Read the model definition and answer for the solid it produces. Units are mm, in the model's axes. Give positions to 0.01 mm unless a question says otherwise; leave off trailing zeros. Order: outer loops, then holes, each group sorted by start corner. A loop starts at its lowest first (then second) coordinate and runs counter-clockwise, first axis right, second up. Notation, with made-up numbers: (-34.75, 83.5) - (-5.75, 83.5) arc R7 cw to (-5.75, 91.5) - close; hole circle Ø7 at (-2, 30). An arc over 180 degrees is marked (long way). Write item = value, one per line.
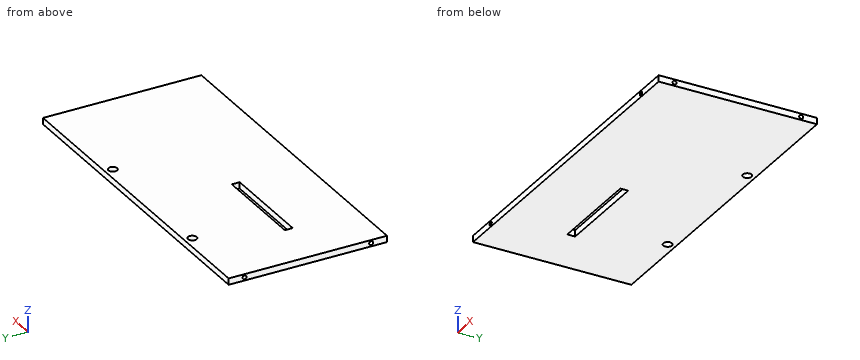
```python
from build123d import *

# Parameters (mm, degrees)
SKETCH_1_W             = 200
SKETCH_1_H             = 100
EXTRUDE_1_DEPTH        = 4
SKETCH_5_R             = 2.75
CUT_EXTRUDE_1_DEPTH    = 5
SKETCH_6_W             = 4
SKETCH_6_H             = 100
EXTRUDE_2_DEPTH        = 10
SKETCH_7_W             = 60
SKETCH_7_H             = 5
CUT_EXTRUDE_2_DEPTH    = 5
HOLE_WIZARD_M3_1_D     = 2.5
HOLE_WIZARD_M3_1_DEPTH = 7.5
HOLE_WIZARD_M3_1_TIP   = 0.751075774
HOLE_WIZARD_M3_2_D     = 2.5
HOLE_WIZARD_M3_2_DEPTH = 7.5
HOLE_WIZARD_M3_2_TIP   = 0.751075774
HOLE_WIZARD_M3_3_D     = 2.5
HOLE_WIZARD_M3_3_DEPTH = 7.5
HOLE_WIZARD_M3_3_TIP   = 0.751075774


with BuildPart() as part:
    # 草图1 → 凸台-拉伸1 (new body)
    with BuildSketch(Plane.XY):
        with Locations((100, 50)):
            Rectangle(SKETCH_1_W, SKETCH_1_H)
    extrude(amount=EXTRUDE_1_DEPTH)

    # 草图5 → 切除-拉伸1 (cut, through all)
    with BuildSketch(Plane(origin=(0, 0, 0), x_dir=(-1, 0, 0), z_dir=(0, 0, -1))):
        with Locations((-50, 95)):
            Circle(SKETCH_5_R)
        with Locations((-140, 95)):
            Circle(SKETCH_5_R)
    extrude(amount=-CUT_EXTRUDE_1_DEPTH, mode=Mode.SUBTRACT)

    # 草图6 → 凸台-拉伸2 (add)
    with BuildSketch(Plane(origin=(200, 0, 0), x_dir=(0, 0, -1), z_dir=(1, 0, 0))):
        with Locations((-2, 50)):
            Rectangle(SKETCH_6_W, SKETCH_6_H)
    extrude(amount=EXTRUDE_2_DEPTH)

    # 草图7 → 切除-拉伸2 (cut)
    with BuildSketch(Plane(origin=(0, 0, 0), x_dir=(-1, 0, 0), z_dir=(0, 0, -1))):
        with Locations((-63, 43.6)):
            Rectangle(SKETCH_7_W, SKETCH_7_H)
    extrude(amount=-CUT_EXTRUDE_2_DEPTH, mode=Mode.SUBTRACT)

    # M3 螺纹孔1
    with Locations(Plane.ZY):
        with Locations((2, 10), (2, 90)):
            Hole(HOLE_WIZARD_M3_1_D / 2, depth=HOLE_WIZARD_M3_1_DEPTH)
            with Locations((0, 0, -(HOLE_WIZARD_M3_1_DEPTH + HOLE_WIZARD_M3_1_TIP / 2))):  # 118° drill point
                Cone(0, HOLE_WIZARD_M3_1_D / 2, HOLE_WIZARD_M3_1_TIP, mode=Mode.SUBTRACT)

    # M3 螺纹孔2
    with Locations(Plane(origin=(210, 0, 0), x_dir=(0, 0, -1), z_dir=(1, 0, 0))):
        with Locations((-2, 10), (-2, 90)):
            Hole(HOLE_WIZARD_M3_2_D / 2, depth=HOLE_WIZARD_M3_2_DEPTH)
            with Locations((0, 0, -(HOLE_WIZARD_M3_2_DEPTH + HOLE_WIZARD_M3_2_TIP / 2))):  # 118° drill point
                Cone(0, HOLE_WIZARD_M3_2_D / 2, HOLE_WIZARD_M3_2_TIP, mode=Mode.SUBTRACT)

    # M3 螺纹孔3
    with Locations(Plane(origin=(0, 0, 0), x_dir=(-1, 0, 0), z_dir=(0, -1, 0))):
        with Locations((-20, -2), (-190, -2)):
            Hole(HOLE_WIZARD_M3_3_D / 2, depth=HOLE_WIZARD_M3_3_DEPTH)
            with Locations((0, 0, -(HOLE_WIZARD_M3_3_DEPTH + HOLE_WIZARD_M3_3_TIP / 2))):  # 118° drill point
                Cone(0, HOLE_WIZARD_M3_3_D / 2, HOLE_WIZARD_M3_3_TIP, mode=Mode.SUBTRACT)


solid = part.part
```
1. Straight lines are drawn through the part: L1, parallel to Y at x = 6.25, z = 2; L2, parallel to Y at x = 37.5, z = 2.6; L3, parallel to Z at x = 3, y = 10. For each, find the intervals that lie inside material, in ascending order. Write a range as [from, to].
Recorded:
L1 = [0, 8.75], [11.25, 88.75], [91.25, 100]
L2 = [0, 41.1], [46.1, 100]
L3 = [0, 0.75], [3.25, 4]
2. Section C-C (y = 95) is taken. Determine the outline of the cut face in (x, z).
Recorded:
outline = (0, 0) - (47.25, 0) - (47.25, 4) - (0, 4) - close; (52.75, 0) - (137.25, 0) - (137.25, 4) - (52.75, 4) - close; (142.75, 0) - (210, 0) - (210, 4) - (142.75, 4) - close
3. Section D-D (z = 1.35) is taken. Count the separate pieces of the cut face and the enclosed holes in it, and give its area (3 significant figures).
Recorded:
separate_pieces = 1
enclosed_holes = 3
area = 20,600 mm^2
4. Flat-ended cylindrical pins translate along their axes: pin 1 (8 mm diameter, centred on x = 172.5, y = 43, fed in from -Z); pin 2 (2 mm diameter, centred on y = 10, z = 2, fed in from +X); pin 3 (2 mm diameter, centred on y = 10, z = 2, fed in from -X); pin 4 (1.5 mm diameter, centred on x = 190, z = 2, fed in from -Y). Find the tip coordinate at first contact, or state that the pin passes through.
Recorded:
pin_1 = 0
pin_2 = 202.35
pin_3 = 7.65
pin_4 = 7.8
5. Section B-B (x = 50) is taken. Determine the outline of the cut face in (y, z), and give its area (3 significant figures).
Recorded:
outline = (0, 0) - (41.1, 0) - (41.1, 4) - (0, 4) - close; (46.1, 0) - (92.25, 0) - (92.25, 4) - (46.1, 4) - close; (97.75, 0) - (100, 0) - (100, 4) - (97.75, 4) - close
area = 358 mm^2
6. Section A-A (x = 72) is taken. Determine the outline of the cut face in (y, z), and give its area (3 significant figures).
Recorded:
outline = (0, 0) - (41.1, 0) - (41.1, 4) - (0, 4) - close; (46.1, 0) - (100, 0) - (100, 4) - (46.1, 4) - close
area = 380 mm^2
